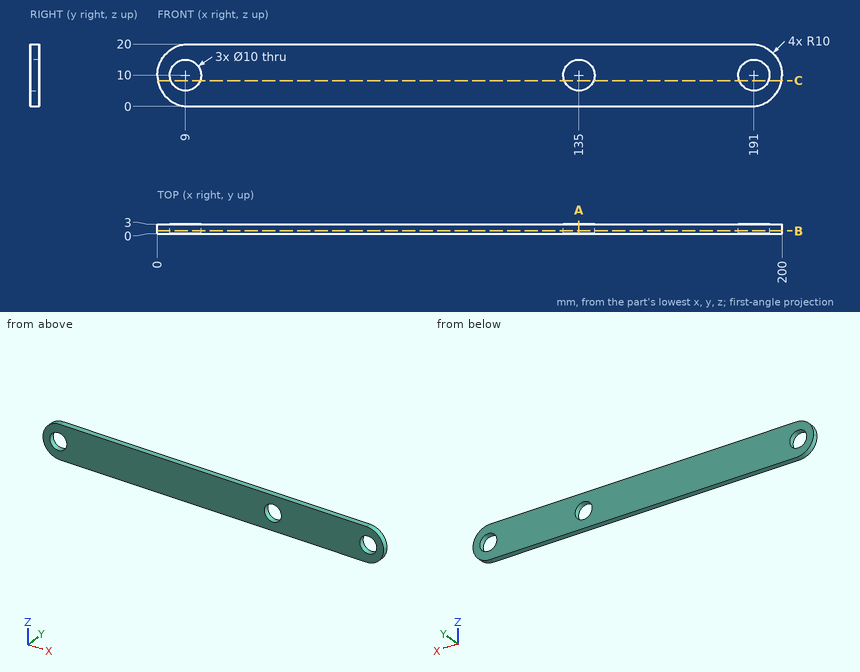
The figure shows three views and two pictorial views of one solid part (mm, origin at its lowest corner). Answer the questions. Give positions to 0.01 mm unless a question says otherwise; leave off trailing zeros. Loops run counter-clockwise (first coordinate to the right, second up) from the corner with the lowest first, then second, coordinate; pieces in that order, holes last. Notation, with made-up numbers: (55.25, 16.25) -> (64.25, 16.25) arc R25 cw to (64.25, 37.25) -> close; hole circle Ø6 at (37.25, 58). An arc over 180 degrees is marked (long way). Use a Markdown table: item, result. Add a question column.
1. Section A-A on x = 135 is taken. Determine the outline of the cut face in (y, z), and give its area (3 significant figures).
2. Find the intervals of material crossed by probe 1 along X at (y, z) = (1.75, 10); probe 2 along X at (y, z) = (2.65, 14) (1 decimal); probe 3 along Z at (x, y) = (131, 2.75), in increasing order.
3. Section B-B on y = 0.95 is taken. State how many separate pieces and enclosed holes the cut face has, and give its area (3 significant figures).
4. Section C-C on z = 8.25 is taken. Determine the outline of the cut face in (x, y), and give its area (3 significant figures).
Results below:
| question | item | result |
|---|---|---|
| 1 | outline | (0, 0) -> (3, 0) -> (3, 5) -> (0, 5) -> close; (0, 15) -> (3, 15) -> (3, 20) -> (0, 20) -> close |
| 1 | area | 30.0 mm^2 |
| 2 | probe 1 | x = 0 to 4, 14 to 130, 140 to 186, 196 to 200 |
| 2 | probe 2 | x = 0.8 to 6, 12 to 132, 138 to 188, 194 to 199.2 |
| 2 | probe 3 | z = 0 to 7, 13 to 20 |
| 3 | separate pieces | 1 |
| 3 | enclosed holes | 3 |
| 3 | area | 3,680 mm^2 |
| 4 | outline | (0.15, 0) -> (4.32, 0) -> (4.32, 3) -> (0.15, 3) -> close; (13.68, 0) -> (130.32, 0) -> (130.32, 3) -> (13.68, 3) -> close; (139.68, 0) -> (186.32, 0) -> (186.32, 3) -> (139.68, 3) -> close; (195.68, 0) -> (199.85, 0) -> (199.85, 3) -> (195.68, 3) -> close |
| 4 | area | 515 mm^2 |
